Build history of the part. All positions in model axes, mm. Face numbers are marked on the shaded views. Give positions to 0.01 mm unless a question says otherwise; leave off trailing zeros. Loops run counter-clockwise (first coordinate to the right, second up) from the corner with the lowest first, then second, coordinate; pieces in that order, holes last. Notation, with made-up numbers: (8, 68) - (29, 68) arc R21 cw to (29, 83) - close; hole circle Ø7 at (49.25, 38). An arc over 180 degrees is marked (long way). Return JSON: item names as keys, results as strings. Group by question number.
1) Slice it at C-C (y = -13.5). List the corners of the cut face in (x, z), and give its area (3 significant figures).
2) Drop flat-ended pins along their axis: pin 1 (4 mm diameter, centred on y = -10.5, z = -3, fed in from -X); pin 2 (3 mm diameter, centred on y = -3.5, z = 4.5, fed in from +X). Give the stop position or say it passes through.
3) Mould opens along Z. For the marked faces 1, 2 and 3 say: released by +Z, released by -Z, zero draft, split by the parting line, or undercut.
4) Slice it at B-B (x = 0). List the corners of the cut face in (y, z).
5) Drill centre lines: probe 1 along Z at (x, y) = (0, -5.5); probe 2 along X at (y, z) = (-10.5, 0.75); probe 3 along X at (y, z) = (-15, -1.25). Where is each one in solid material? Low to high. Write a range as from..to.
6) Slice it at A-A (z = 0). List the corners of the cut face in (x, y), and give its area (3 significant figures).
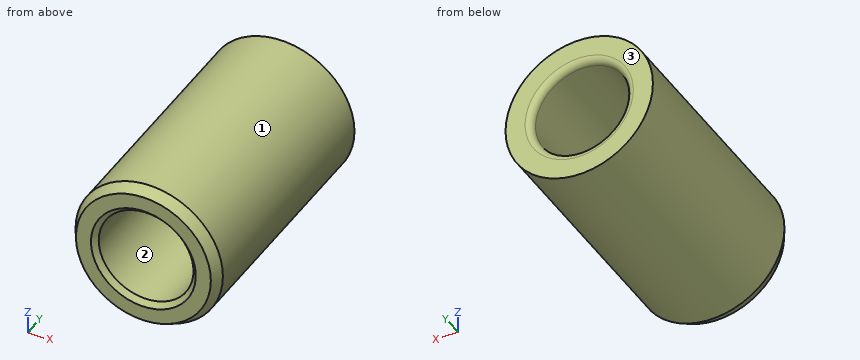
```python
from build123d import *

# Parameters (mm, degrees)
CHAMFER1_SIZE  = 0.8128
CHAMFER1_SIZE2 = 0.469270299


with BuildPart() as part:
    # Sketch1 → BODY (revolve)
    with BuildSketch(Plane.XY, mode=Mode.PRIVATE) as body_sk:
        with BuildLine():
            Line((4.079875, 0), (5.55625, 0))
            Line((5.55625, 0), (5.55625, -19.05))
            Line((5.55625, -19.05), (3.952875, -19.05))
            Line((3.952875, -19.05), (3.571875, -18.669))
            Line((3.571875, -18.669), (3.571875, -0.508))
            ThreePointArc((3.571875, -0.508), (3.720664755, -0.148789755), (4.079875, 0))
        make_face()
    revolve(body_sk.sketch.rotate(Axis((0, 0, 0), (0, -1, 0)), 180), axis=Axis((0, 0, 0), (0, -1, 0)))

    # Chamfer1
    chamfer1_edges = [part.edges().sort_by_distance(p)[0] for p in [
        (5.55625, -19.05, 0),
    ]]
    chamfer1_side = [part.faces().sort_by_distance(p)[0] for p in [
        (5.55625, -9.525, 0),
    ]]
    chamfer(chamfer1_edges, length=CHAMFER1_SIZE, length2=CHAMFER1_SIZE2, reference=chamfer1_side[0])


solid = part.part
```
Results:
{
 "1": {"outline": "circle Ø11.11 at (0, 0); hole circle Ø7.14 at (0, 0)", "area": "56.9 mm2"},
 "2": {"pin 1": "x = -5.47", "pin 2": "x = 4.68"},
 "3": {"face 1": "split by the parting line", "face 2": "undercut", "face 3": "zero draft"},
 "4": {"outline": "(-19.05, -5.09) - (-18.24, -5.56) - (0, -5.56) - (0, -4.08) arc R0.51 ccw to (-0.51, -3.57) - (-18.67, -3.57) - (-19.05, -3.95) - close; (-19.05, 3.95) - (-18.67, 3.57) - (-0.51, 3.57) arc R0.51 ccw to (0, 4.08) - (0, 5.56) - (-18.24, 5.56) - (-19.05, 5.09) - close"},
 "5": {"probe 1": "-5.56..-3.57, 3.57..5.56", "probe 2": "-5.51..-3.49, 3.49..5.51", "probe 3": "-5.41..-3.35, 3.35..5.41"},
 "6": {"outline": "(-5.56, -18.24) - (-5.09, -19.05) - (-3.95, -19.05) - (-3.57, -18.67) - (-3.57, -0.51) arc R0.51 ccw to (-4.08, 0) - (-5.56, 0) - close; (3.57, -18.67) - (3.95, -19.05) - (5.09, -19.05) - (5.56, -18.24) - (5.56, 0) - (4.08, 0) arc R0.51 ccw to (3.57, -0.51) - close", "area": "75.0 mm2"}
}
